Read the model definition and answer for the solid it produces. Units are mm, in the model's axes. A direction names the side the tool comes from. Give positions to 0.01 mm unless a question says otherwise; leave off trailing zeros. Loops run counter-clockwise (first coordinate to the right, second up) from the corner with the lowest first, then second, coordinate; pieces in that order, holes last. Notation, with made-up numbers: (51, 89) - (66, 89) arc R23 cw to (66, 105) - close; hole circle Ø6 at (11.25, 60). An arc over 180 degrees is marked (long way). Put each result on its own line as item: value. Start each with the question number.
1. Given pin 1 Ø6 at (x, z) = (-237, -145) entering from -Y; pin 2 Ø5.5 at (x, y) = (-55, 113.5) entering from -Z; pin 3 Ø1.5 at (x, y) = (-117.5, 113.5) entering from +Z; pin 4 Ø1 at (x, z) = (-203.5, -216) entering from +Y, each flat-ended and moving along its own axis, determine where each tip first touches the part or whether it passes through.
2. A cutting plane is placed at A-A, the plane x = 0. Determine the outline of the cut face in (y, z).
3. A cutting plane is placed at B-B, the plane y = 55.5. Determine the outline of the cut face in (x, z), plus the area to 3 significant figures.
4. A cutting plane is placed at C-C, the plane z = -151. Determine the outline of the cut face in (x, y).
5. A cutting plane is placed at D-D, the plane x = -331.5. Determine the outline of the cut face in (y, z).
6. For faces 4 (the cylindrical face through (206.517, 112.465, -239.222)), 5 (the cylindrical face through (12.015, 116.041, -191.847)), 6 (the flat face through (186.324, 112.465, -308.578)), determine the directions among +Z, -Z, +X, -X, +Y, -Y from which every point of the face is accessible in a straight line to the end or side of a thin tool.
7. For a pull along Y with two mould halves and no side action, classify faces 1 (the cylindrical face through (3.83, 114.93, -239.237)), 2 (the flat face through (-6, 0, -6)), 3 (the cylindrical face through (-127.66, 59.3, -331.525)) as released by +Y, released by -Y, zero draft, split by the parting line, or undercut.
8. Consider L1, parallel to X at y = 116.25, z = -230; L2, parallel to Y at x = -108.5, z = 139; L3, parallel to Y at x = -20, z = -273. Determine where each line is inside the solid, lowest interval first. Write a range as from..to.
```python
from build123d import *

# Parameters (mm, degrees)
SKETCH1_W                = 800
SKETCH1_H                = 800
BOSS_EXTRUDE4_DEPTH      = 10
SKETCH6_R                = 20
BOSS_EXTRUDE5_DEPTH      = 100
BOSS_EXTRUDE6_DEPTH      = 5
BOSS_EXTRUDE7_DEPTH      = 5
BOSS_EXTRUDE7_DEPTH_BACK = 5
SKETCH8_R                = 40
CUT_EXTRUDE1_DEPTH       = 5
CUT_EXTRUDE1_DEPTH_BACK  = 24
SKETCH9_R                = 10


with BuildPart() as part:
    # Sketch1 → Boss-Extrude4 (new body)
    with BuildSketch(Plane(origin=(0, 0, 0), x_dir=(1, 0, 0), z_dir=(0, 1, 0))):
        Rectangle(SKETCH1_W, SKETCH1_H)
    extrude(amount=BOSS_EXTRUDE4_DEPTH)

    # Sketch6 → Boss-Extrude5 (add)
    with BuildSketch(Plane(origin=(0, 10, 0), x_dir=(1, 0, 0), z_dir=(0, 1, 0))):
        with Locations(Location((120, 350, 0), (0, 0, 270))):
            Circle(SKETCH6_R)
        with Locations(Location((-120, 350, 0), (0, 0, 270))):
            Circle(SKETCH6_R)
        with Locations(Location((-180, 250, 0), (0, 0, 270))):
            Circle(SKETCH6_R)
        with Locations(Location((180, 250, 0), (0, 0, 270))):
            Circle(SKETCH6_R)
    extrude(amount=BOSS_EXTRUDE5_DEPTH)

    # Sketch7 → Boss-Extrude6 (add)
    with BuildSketch(Plane(origin=(0, 110, 0), x_dir=(1, 0, 0), z_dir=(0, 1, 0))):
        with BuildLine():
            Line((-120, 370), (120, 370))
            Line((120, 370), (146.81207684, 370))
            ThreePointArc((146.81207684, 370), (157.821897015, 366.696821845), (165.194977441, 357.878385972))
            Line((165.194977441, 357.878385972), (208.052120298, 257.878385972))
            ThreePointArc((208.052120298, 257.878385972), (206.366041542, 238.990179825), (189.669219698, 230))
            Line((189.669219698, 230), (180, 230))
            Line((180, 230), (-180, 230))
            Line((-180, 230), (-189.669219698, 230))
            ThreePointArc((-189.669219698, 230), (-206.366041542, 238.990179825), (-208.052120298, 257.878385972))
            Line((-208.052120298, 257.878385972), (-165.194977441, 357.878385972))
            ThreePointArc((-165.194977441, 357.878385972), (-157.821897015, 366.696821845), (-146.81207684, 370))
            Line((-146.81207684, 370), (-120, 370))
        make_face()
    extrude(amount=BOSS_EXTRUDE6_DEPTH)

    # Sketch8 → Boss-Extrude7 (add, two sides: drawn at the far end of the back side and taken through both)
    with BuildSketch(Plane(origin=(0, 115, 0), x_dir=(1, 0, 0), z_dir=(0, 1, 0)).offset(-BOSS_EXTRUDE7_DEPTH_BACK)):
        with Locations(Location((0, 230, 0), (0, 0, 270))):
            Circle(SKETCH8_R)
    extrude(amount=BOSS_EXTRUDE7_DEPTH + BOSS_EXTRUDE7_DEPTH_BACK)

    # Sketch9 → Cut-Extrude1 (cut, two sides: drawn at the far end of the back side and taken through both)
    with BuildSketch(Plane(origin=(0, 120, 0), x_dir=(1, 0, 0), z_dir=(0, 1, 0)).offset(-CUT_EXTRUDE1_DEPTH_BACK)):
        with Locations(Location((0, 230, 0), (0, 0, 90))):
            Circle(SKETCH9_R)
    extrude(amount=CUT_EXTRUDE1_DEPTH + CUT_EXTRUDE1_DEPTH_BACK, mode=Mode.SUBTRACT)


solid = part.part
```
Return value:
1. pin 1: stops at y = 0
1. pin 2: stops at z = -370
1. pin 3: stops at z = -230
1. pin 4: stops at y = 10
2. outline: (0, -400) - (10, -400) - (10, 400) - (0, 400) - close; (110, -370) - (115, -370) - (115, -270) - (120, -270) - (120, -240) - (110, -240) - close; (110, -220) - (120, -220) - (120, -190) - (110, -190) - close
3. outline: circle Ø40 at (-180, -250); circle Ø40 at (-120, -350); circle Ø40 at (120, -350); circle Ø40 at (180, -250)
3. area: 5,030 mm2
4. outline: (-400, 0) - (400, 0) - (400, 10) - (-400, 10) - close
5. outline: (0, -400) - (10, -400) - (10, 400) - (0, 400) - close
6. face 4: +X, +Y
6. face 5: +Y
6. face 6: -Z, +X, +Y
7. face 1: zero draft
7. face 2: released by -Y
7. face 3: undercut
8. L1: x = -40..-10, 10..40
8. L2: y = 0..10
8. L3: y = 0..10, 110..115
